```python
from build123d import *

# Parameters (mm, degrees)
BOARD_DEPTH            = 1.6
BOARDSKETCH_3_R        = 2.54
BOARD_HOLES_DEPTH      = 1.6
PORT_SKETCH_W          = 14.4
PORT_SKETCH_H          = 9
BARREL_CONN_DEPTH      = 11
BARREL_SKETCH_R        = 3.25
BARREL_CONN_HOLE_DEPTH = 9
PORTSKETCH_3_W         = 10.16
PORTSKETCH_3_H         = 2.54
PIN_HEADER_DEPTH       = 7.5
PORTSKETCH_4_W         = 57
PORTSKETCH_4_H         = 30.5
ESP8266_DEPTH          = 4
USB_SKETCH_W           = 5
USB_SKETCH_H           = 10
USB_PORT_DEPTH         = 3
LM7805_SKETCH_W        = 4.64
LM7805_SKETCH_H        = 10.24
LM7805_TH_DEPTH        = 9.07


with BuildPart() as part:
    # Board_Sketch → Board (new body)
    with BuildSketch(Plane(origin=(0, 0, 0), x_dir=(1, 0, 0), z_dir=(0, 1, 0))):
        with BuildLine():
            Line((30.48, -36.83), (30.48, 16.51))
            ThreePointArc((30.48, 16.51), (30.286654013, 17.482015918), (29.736051224, 18.306051224))
            Line((29.736051224, 18.306051224), (9.416051224, 38.626051224))
            ThreePointArc((9.416051224, 38.626051224), (8.592015918, 39.176654013), (7.62, 39.37))
            Line((7.62, 39.37), (-27.94, 39.37))
            ThreePointArc((-27.94, 39.37), (-29.736051224, 38.626051224), (-30.48, 36.83))
            Line((-30.48, 36.83), (-30.48, -36.83))
            ThreePointArc((-30.48, -36.83), (-29.736051224, -38.626051224), (-27.94, -39.37))
            Line((-27.94, -39.37), (27.94, -39.37))
            ThreePointArc((27.94, -39.37), (29.736051224, -38.626051224), (30.48, -36.83))
        make_face()
    extrude(amount=BOARD_DEPTH)

    # BoardSketch<3> → Board_Holes (cut)
    with BuildSketch(Plane(origin=(0, 0, 0), x_dir=(1, 0, 0), z_dir=(0, 1, 0))):
        with Locations((-25.400144884, -34.290144884)):
            Circle(BOARDSKETCH_3_R)
        with Locations((25.400144884, -34.290144884)):
            Circle(BOARDSKETCH_3_R)
        with Locations((-25.400144884, 34.290144884)):
            Circle(BOARDSKETCH_3_R)
    extrude(amount=BOARD_HOLES_DEPTH, mode=Mode.SUBTRACT)

    # Port_Sketch → Barrel_Conn (add)
    with BuildSketch(Plane(origin=(0, 1.6, 0), x_dir=(1, 0, 0), z_dir=(0, 1, 0))):
        with Locations((-20.737, 24.97)):
            Rectangle(PORT_SKETCH_W, PORT_SKETCH_H)
    extrude(amount=BARREL_CONN_DEPTH)

    # Barrel_Sketch → Barrel_Conn_Hole (cut)
    with BuildSketch(Plane.ZY.offset(27.937)):
        with Locations((-24.97, 8.1)):
            Circle(BARREL_SKETCH_R)
    extrude(amount=-BARREL_CONN_HOLE_DEPTH, mode=Mode.SUBTRACT)

    # PortSketch<3> → Pin_Header (add)
    with BuildSketch(Plane(origin=(0, 1.6, 0), x_dir=(1, 0, 0), z_dir=(0, 1, 0))):
        with Locations((22.86, -26.67)):
            Rectangle(PORTSKETCH_3_W, PORTSKETCH_3_H)
    extrude(amount=PIN_HEADER_DEPTH)

    # PortSketch<4> → ESP8266 (add)
    with BuildSketch(Plane(origin=(0, 1.6, 0), x_dir=(1, 0, 0), z_dir=(0, 1, 0))):
        with Locations((-0.48, -7.61)):
            Rectangle(PORTSKETCH_4_W, PORTSKETCH_4_H)
    extrude(amount=ESP8266_DEPTH)

    # USB_Sketch → USB_Port (add)
    with BuildSketch(Plane(origin=(0, 5.6, 0), x_dir=(1, 0, 0), z_dir=(0, 1, 0))):
        with Locations((-26.48, -7.61)):
            Rectangle(USB_SKETCH_W, USB_SKETCH_H)
    extrude(amount=USB_PORT_DEPTH)

    # LM7805_Sketch → LM7805_TH (add)
    with BuildSketch(Plane.XZ):
        with Locations((-1.685, -5.04)):
            Rectangle(LM7805_SKETCH_W, LM7805_SKETCH_H)
    extrude(amount=LM7805_TH_DEPTH)


solid = part.part
```
Check sheet for the modelled part. Datum: model origin and axes. Units: mm. A direction names the side the tool comes from. Round coordinates to 2 decimals unless told otherwise and drop trailing zeros. Loops run counter-clockwise (first coordinate to the right, second up) from the corner with the lowest first, then second, coordinate; pieces in that order, holes last. Notation, with made-up numbers: (26, -3) - (80, -3) arc R32 ccw to (80, 27) - close; hole circle Ø10 at (43, -39). An arc over 180 degrees is marked (long way). Answer as a JSON object with one key per item and string values. Group by question number.
Q1. Sectioned sample at D-D, the plane z = -24.97. Enter the section's corners in (x, y).
Q2. Sectioned sample at B-B, the plane z = 7. Enter the section's corners in (x, y).
Q3. Mould release check, pull along Z, two halves, no side actions. Record for faces 6 (the face through (-7, 0, -1)), 7 (the face through (-24.03, 0.79, -36.43)), 8 (the face through (-2, -4, 0.08)): released by +Z, released by -Z, zero draft, split by the parting line, or undercut.
Q4. Set-up check for faces 1 (the face through (17.78, 5, 27)), 2 (the face through (-27, 7, 2.61)), 3 (the face through (-27, 7, 12.61)), 4 (the face through (-28.98, 4, 8)), 5 (the face through (-2, -4, -10.16)): record each of +Z, -Z, +X, -X, +Y, -Y from which the full face is reachable in a straight line by a thin tool's end or side.
Q5. Gauge pin test, flat ends, axial feed: P1, Ø6, axis at x = 9, z = 18, coming from the +Y side; P2, Ø4, axis at y = 7, z = 12, coming from the -X side; P3, Ø2.5, axis at x = -26, y = 7, coming from the -Z side. Record the tip position at first contact, or that the pin passes through.
Q6. Scan lines: line 1 along Y through (x, z) = (15, -28); line 2 along Y through (x, z) = (-17, -2); line 3 along Z through (x, y) = (6, 2.5). Record each from-to range of solid material in increasing order. Write a range as [from, to].
Q7. Sectioned sample at A-A, the plane x = 6. Enter the section's corners in (y, z).
Q8. Sectioned sample at C-C, the plane y = -4. Enter the section's corners in (x, z) (3 decimals), plus the area to 3 significant figures.
Solution:
{
 "1": {"outline": "(-30.48, 0) - (23.07, 0) - (23.07, 1.6) - (-13.54, 1.6) - (-13.54, 12.6) - (-27.94, 12.6) - (-27.94, 11.35) - (-18.94, 11.35) - (-18.94, 4.85) - (-27.94, 4.85) - (-27.94, 1.6) - (-30.48, 1.6) - close"},
 "2": {"outline": "(-30.48, 0) - (30.48, 0) - (30.48, 1.6) - (28.02, 1.6) - (28.02, 5.6) - (-23.98, 5.6) - (-23.98, 8.6) - (-28.98, 8.6) - (-28.98, 1.6) - (-30.48, 1.6) - close"},
 "3": {"face 6": "zero draft", "face 7": "undercut", "face 8": "released by +Z"},
 "4": {"face 1": "+Z, -X, +Y", "face 2": "+X, -X, +Y", "face 3": "+Z, +X, -X, +Y", "face 4": "+Z, -Z, -X, +Y", "face 5": "-Z, +X, -X, -Y"},
 "5": {"P1": "stops at y = 5.6", "P2": "stops at x = -28.98", "P3": "stops at z = -29.47"},
 "6": {"line 1": "y = [0, 1.6]", "line 2": "y = [0, 5.6]", "line 3": "z = [-7.64, 22.86]"},
 "7": {"outline": "(0, -39.37) - (1.6, -39.37) - (1.6, -7.64) - (5.6, -7.64) - (5.6, 22.86) - (1.6, 22.86) - (1.6, 39.37) - (0, 39.37) - close"},
 "8": {"outline": "(-4.005, -10.16) - (0.635, -10.16) - (0.635, 0.08) - (-4.005, 0.08) - close", "area": "47.5 mm²"}
}
